Drawing for the job (mm, zero at the part's lowest x, y, z). A direction names the side the tool comes from. Coordinates: 2 decimals unless noted, no trailing zeros. Order: outer loops, then holes, each group sorted by start corner. A loop starts at its lowest first (then second) coordinate and runs counter-clockwise, first axis right, second up.
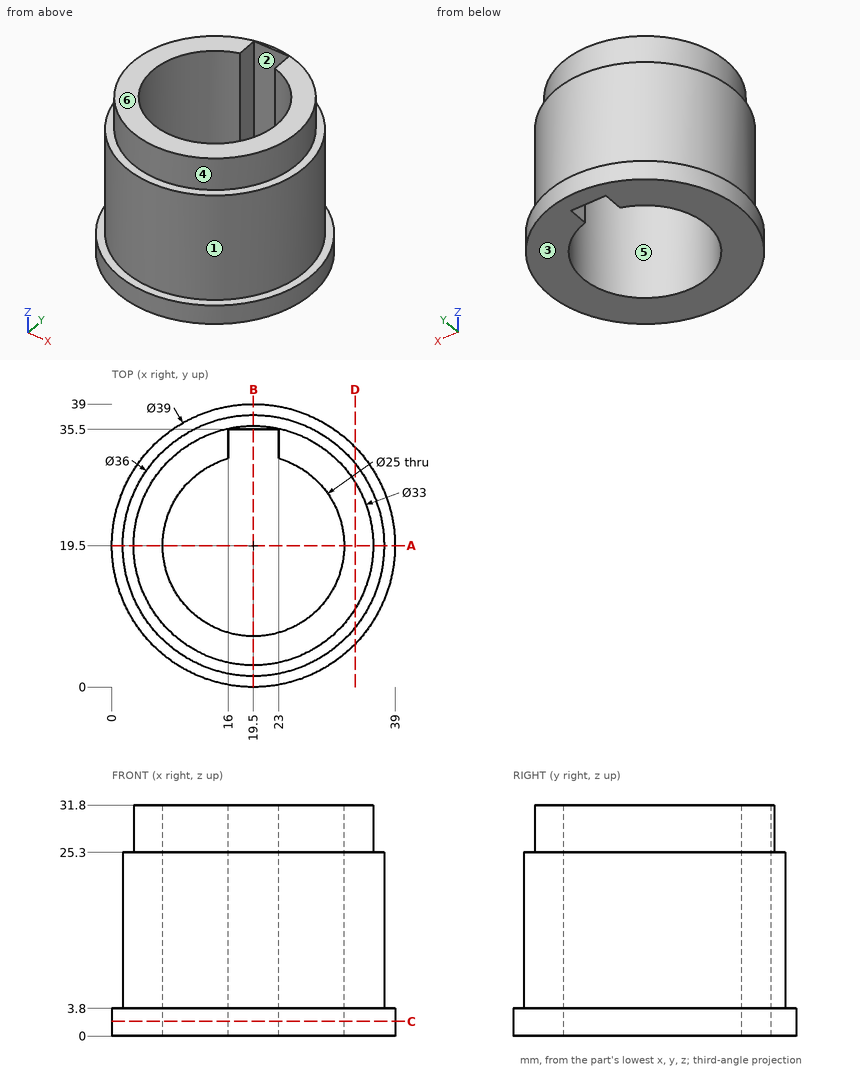
1) Slice it at B-B (x = 19.5). List the corners of the cut face in (y, z), plus the area to 3 significant figures.
2) Slice it at C-C (z = 2). List the corners of the cut face in (x, y).
3) Slice it at A-A (y = 19.5). List the corners of the cut face in (x, z), plus the area to 3 significant figures.
4) Drill centre lines: probe 1 along Y at (x, z) = (19, 23); probe 2 along X at (y, z) = (19, 17); probe 3 along Y at (x, z) = (24, 6.5). Where is each one in solid material? Low to high.
5) Slice it at D-D (x = 33.5). List the corners of the cut face in (y, z), plus the area to 3 significant figures.
6) Which spindle directions (+Z, -Z, +X, -X, +Y, -Y) get a long thin tool onto all of the face, cutting with end or side? Do the marked faces 1, 2 and 3. Say none if no direction does.
7) Pin check, flat tips, straight feed: P1, Ø1.5, axis at x = 33.5, z = 11, coming from the -Y side; P2, Ø1.2, axis at y = 34, z = 11.5, coming from the +X side; P3, Ø1, axis at y = 27, z = 17.5, coming from the +X side; P4, Ø11.5, axis at x = 23.5, y = 24, coming from the +Z side. Stop position of each tip, or through.
8) Two-plate mould, pull along X, no slides. Class the marked faces 4, 5 and 6: released by +X, released by -X, zero draft, split by the parting line, or undercut.
Worked out:
1. outline: (0, 0) - (7, 0) - (7, 31.8) - (3, 31.8) - (3, 25.3) - (1.5, 25.3) - (1.5, 3.8) - (0, 3.8) - close; (35.5, 0) - (39, 0) - (39, 3.8) - (37.5, 3.8) - (37.5, 25.3) - (36, 25.3) - (36, 31.8) - (35.5, 31.8) - close
1. area: 230 mm2
2. outline: circle Ø39 at (19.5, 19.5); hole (16, 31.5) arc R12.5 ccw (long way) to (23, 31.5) - (23, 35.5) - (16, 35.5) - close
3. outline: (0, 0) - (7, 0) - (7, 31.8) - (3, 31.8) - (3, 25.3) - (1.5, 25.3) - (1.5, 3.8) - (0, 3.8) - close; (32, 0) - (39, 0) - (39, 3.8) - (37.5, 3.8) - (37.5, 25.3) - (36, 25.3) - (36, 31.8) - (32, 31.8) - close
3. area: 342 mm2
4. probe 1: y = 1.51 to 7.01, 35.5 to 37.49
4. probe 2: x = 1.51 to 7.01, 31.99 to 37.49
4. probe 3: y = 2.07 to 7.84, 31.16 to 36.93
5. outline: (5.93, 0) - (33.07, 0) - (33.07, 3.8) - (30.81, 3.8) - (30.81, 25.3) - (28.23, 25.3) - (28.23, 31.8) - (10.77, 31.8) - (10.77, 25.3) - (8.19, 25.3) - (8.19, 3.8) - (5.93, 3.8) - close
5. area: 703 mm2
6. face 1: +Z
6. face 2: +Z, -Z
6. face 3: -Z, +X, -X, +Y, -Y
7. P1: stops at y = 7.32
7. P2: stops at x = 30.94
7. P3: stops at x = 36.08
7. P4: passes through
8. face 4: split by the parting line
8. face 5: undercut
8. face 6: zero draft
